Autodesk Inventor part; units mm, degrees
ref_plane "YZ Plane" through (0, 0, 0) normal (1, 0, 0) x (0, 1, 0)
ref_plane "XZ Plane" through (0, 0, 0) normal (0, 1, 0) x (-1, 0, 0)
ref_plane "XY Plane" through (0, 0, 0) normal (0, 0, 1) x (1, 0, 0)
sketch "Sketch1" plane through (0, 0, 0) normal (0, 1, 0) x (-1, 0, 0)
  line L0 (-12.7, -148.5) -> (12.7, -148.5)
  line L1 (12.7, -148.5) -> (12.7, 148.5)
  line L2 (12.7, 148.5) -> (-12.7, 148.5)
  line L3 (-12.7, 148.5) -> (-12.7, -148.5)
  line L4 (-12.7, -148.5) -> (12.7, 148.5) construction
  line L5 (12.7, -148.5) -> (-12.7, 148.5) construction
  point P0 (0, 0)
  dimension "d0" = 25.4
  dimension "d1" = 297
extrude "Extrusion1" add sketch "Sketch1" along normal blind 10
sketch "Sketch2" plane through (0, 0, 0) normal (0, -1, 0) x (1, 0, 0)
  line L0 (12.7, -148.5) -> (-12.7, -148.5)
  line L1 (12.7, 148.5) -> (12.7, -148.5)
  line L2 (-12.7, 148.5) -> (12.7, 148.5)
  line L3 (-12.7, -148.5) -> (-12.7, 148.5)
  line L4 (17.7, -153.5) -> (-17.7, -153.5)
  line L5 (-17.7, -153.5) -> (-17.7, 153.5)
  line L6 (-17.7, 153.5) -> (17.7, 153.5)
  line L7 (17.7, 153.5) -> (17.7, -153.5)
  point P0 (0, 0)
  dimension "d4" = 5
extrude "Extrusion2" add sketch "Sketch2" along normal blind 3 contours L0 L3 L2 L1 | L4 L5 L6 L7
sketch "Sketch3" plane through (0, 10, 0) normal (0, 1, 0) x (1, 0, 0)
  line L0 (12.7, 148.5) -> (-12.7, 148.5)
  line L1 (-12.7, 148.5) -> (-12.7, -148.5)
  line L2 (-12.7, -148.5) -> (12.7, -148.5)
  line L3 (12.7, -148.5) -> (12.7, 148.5)
  circle A0 centre (0, -130) radius 5
  point P0 (0, 0)
  dimension "d7" = 10
  dimension "d8" = 130
extrude "Extrusion3" cut sketch "Sketch3" against normal through all contours A0
fillet "Fillet1" radius 1 8 edges at (12.7, 5, 148.5) (-12.7, 5, 148.5) (12.7, 5, -148.5) (-12.7, 5, -148.5) (0, 10, -148.5) (-12.7, 10, 0) (12.7, 10, 0) (0, 10, 148.5)
properties part number "enclosureTop"
Geometry check sheet. Reference: the model listing, model coordinates, mm. A direction names the side the tool comes from. Round coordinates to 2 decimals unless told otherwise and drop trailing zeros. Loops run counter-clockwise (first coordinate to the right, second up) from the corner with the lowest first, then second, coordinate; pieces in that order, holes last. Notation, with made-up numbers: (-19.5, 58.5) - (37.5, 58.5) arc R19 ccw to (37.5, 69.5) - close; hole circle Ø3 at (-32.5, 64). An arc over 180 degrees is marked (long way). Use a Markdown table: item, result.
Q1. Cross-section at D-D on z = 45.5. Record the cut outline in (x, y).
Solutions:
| item | result |
|---|---|
| outline | (-17.7, -3) - (17.7, -3) - (17.7, 0) - (12.7, 0) - (12.7, 9) arc R1 ccw to (11.7, 10) - (-11.7, 10) arc R1 ccw to (-12.7, 9) - (-12.7, 0) - (-17.7, 0) - close |
Q2. Cross-section at C-C on y = 5.5. Record the cut outline in (x, z).
Solutions:
| item | result |
|---|---|
| outline | (-12.7, -147.5) arc R1 ccw to (-11.7, -148.5) - (11.7, -148.5) arc R1 ccw to (12.7, -147.5) - (12.7, 147.5) arc R1 ccw to (11.7, 148.5) - (-11.7, 148.5) arc R1 ccw to (-12.7, 147.5) - close; hole circle Ø10 at (0, 130) |
Q3. Access from +Z, -Z, +X, -X, +Y, -Y to the whole of each face (thin tool, end or side, straight path). Record for faces 4 (the flat face through (12.7, 4, 2)), 5 (the flat face through (0, 4, -148.5)), 6 (the flat face through (0, -3, 2)).
Solutions:
| item | result |
|---|---|
| face 4 | +Z, -Z, +X, +Y |
| face 5 | -Z, +X, -X, +Y |
| face 6 | +Z, -Z, +X, -X, -Y |
Q4. Go/stop test with flat-tipped pins: P1, Ø3, axis at x = -7.5, y = 5, coming from the +Z side; P2, Ø5, axis at y = 8.5, z = -14, coming from the -X side; P3, Ø4, axis at x = 13.5, y = 7.5, coming from the -Z side; P4, Ø6, axis at x = 0, z = 130, coming from the +Y side. Record where each tip stops, or that it passes through.
Solutions:
| item | result |
|---|---|
| P1 | stops at z = 148.5 |
| P2 | stops at x = -12.7 |
| P3 | stops at z = -148.5 |
| P4 | passes through |
Q5. Draft check along Z on faces 1 (the cylindrical face through (2.307, 3.591, 134.436)), 2 (the flat face through (-12.7, 4, -2)), 3 (the flat face through (0, 4, 148.5)). Enter one of: released by +Z, released by -Z, zero draft, split by the parting line, or undercut.
Solutions:
| item | result |
|---|---|
| face 1 | undercut |
| face 2 | zero draft |
| face 3 | released by +Z |
Q6. Cross-section at B-B on x = 0. Record the cut outline in (y, z), plus the area to 3 significant figures.
Solutions:
| item | result |
|---|---|
| outline | (-3, -153.5) - (0, -153.5) - (0, -148.5) - (9, -148.5) arc R1 ccw to (10, -147.5) - (10, 125) - (-3, 125) - close; (-3, 135) - (10, 135) - (10, 147.5) arc R1 ccw to (9, 148.5) - (0, 148.5) - (0, 153.5) - (-3, 153.5) - close |
| area | 3,760 mm2 |
Q7. Material ranges on line 1 (X direction, y = -0.5, z = 130); line 2 (Z direction, x = 0, y = 0.25); line 3 (X direction, y = 2.5, z = 130), recorded low to high.
Solutions:
| item | result |
|---|---|
| line 1 | x = -17.7 to -5, 5 to 17.7 |
| line 2 | z = -148.5 to 125, 135 to 148.5 |
| line 3 | x = -12.7 to -5, 5 to 12.7 |
Q8. Cross-section at A-A on z = 130. Record the cut outline in (x, y), plus the area to 3 significant figures.
Solutions:
| item | result |
|---|---|
| outline | (-17.7, -3) - (-5, -3) - (-5, 10) - (-11.7, 10) arc R1 ccw to (-12.7, 9) - (-12.7, 0) - (-17.7, 0) - close; (5, -3) - (17.7, -3) - (17.7, 0) - (12.7, 0) - (12.7, 9) arc R1 ccw to (11.7, 10) - (5, 10) - close |
| area | 230 mm2 |
